from build123d import *

# Parameters (mm, degrees)
BASEKEY_DEPTH = 4
CHAMFER1_SIZE = 0.6


with BuildPart() as part:
    # Sketch1 → BaseKey (new, symmetric)
    with BuildSketch(Plane.XY):
        with BuildLine():
            Line((-12, 5), (0, 5))
            ThreePointArc((0, 5), (5, 0), (0, -5))
            Line((0, -5), (-12, -5))
            ThreePointArc((-12, -5), (-17, 0), (-12, 5))
        make_face()
    extrude(amount=BASEKEY_DEPTH, both=True)

    # Chamfer1
    chamfer1_edges = [part.edges().sort_by_distance(p)[0] for p in [
        (5, 0, 4),
        (-6, 5, 4),
        (-17, 0, 4),
        (-6, 5, -4),
        (5, 0, -4),
        (-6, -5, -4),
        (-17, 0, -4),
        (-6, -5, 4),
    ]]
    chamfer(chamfer1_edges, length=CHAMFER1_SIZE)


solid = part.part
The model under review builds one solid part; all positions refer to its coordinate system, in mm. Coordinates: 2 decimals unless noted, no trailing zeros. Loops run counter-clockwise (first coordinate to the right, second up) from the corner with the lowest first, then second, coordinate; pieces in that order, holes last. Notation, with made-up numbers: (38.25, 45) -> (81.25, 45) arc R35 ccw to (81.25, 83) -> close; hole circle Ø8 at (4, 49). An arc over 180 degrees is marked (long way). Use a Markdown table: item, result. Add a question column.
1. Clearance check with a flat-ended pin moving along its axis: pin 1 Ø4 at (y, z) = (2.5, -2.5) entering from +X. State where the tip first meets the part, or that it passes through.
2. To check wall thickness, follow line 1 (X direction, y = 1.25, z = 0); line 2 (X direction, y = 1, z = -2.25); line 3 (Y direction, x = -13.75, z = 1.75). State the ranges of each line that lie inside material, in increasing order.
3. Add section A-A on z = -1.25. Write out the cut boundary in (x, y), plus the area to 3 significant figures.
Returned:
| question | item | result |
|---|---|---|
| 1 | pin 1 | stops at x = 4.97 |
| 2 | line 1 | x = -16.84 to 4.84 |
| 2 | line 2 | x = -16.9 to 4.9 |
| 2 | line 3 | y = -4.68 to 4.68 |
| 3 | outline | (-12, -5) -> (0, -5) arc R5 ccw to (0, 5) -> (-12, 5) arc R5 ccw to start |
| 3 | area | 199 mm² |
